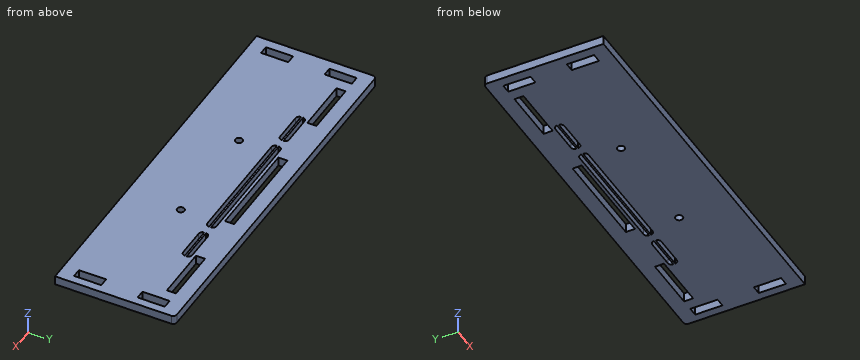
Autodesk Inventor part; units mm, degrees
ref_plane "YZ Plane" through (0, 0, 0) normal (1, 0, 0) x (0, 1, 0)
ref_plane "XZ Plane" through (0, 0, 0) normal (0, 1, 0) x (-1, 0, 0)
ref_plane "XY Plane" through (0, 0, 0) normal (0, 0, 1) x (1, 0, 0)
sketch "Sketch1" plane through (0, 0, 0) normal (0, 0, 1) x (1, 0, 0)
  line L0 (-104.38, -32.9991) -> (103.62, -32.9991)
  line L1 (-102.38, 33.0009) -> (101.62, 33.0009)
  line L2 (57.998, 18.2189) -> (41.998, 18.2189)
  line L3 (41.998, 13.2189) -> (57.998, 13.2189)
  line L4 (-58.002, 18.2189) -> (-42.002, 18.2189)
  line L5 (-42.002, 13.2189) -> (-58.002, 13.2189)
  line L6 (32.998, 18.2189) -> (-33.002, 18.2189)
  line L7 (-33.002, 13.2189) -> (32.998, 13.2189)
  arc A0 (34.998, 16.2189) -> (32.998, 18.2189) centre (32.998, 16.2189) ccw
  arc A1 (-35.002, 15.2189) -> (-33.002, 13.2189) centre (-33.002, 15.2189) ccw
  arc A2 (-33.002, 18.2189) -> (-35.002, 16.2189) centre (-33.002, 16.2189) ccw
  arc A3 (-40.002, 16.2189) -> (-42.002, 18.2189) centre (-42.002, 16.2189) ccw
  arc A4 (-42.002, 13.2189) -> (-40.002, 15.2189) centre (-42.002, 15.2189) ccw
  arc A5 (-60.002, 15.2189) -> (-58.002, 13.2189) centre (-58.002, 15.2189) ccw
  arc A6 (-58.002, 18.2189) -> (-60.002, 16.2189) centre (-58.002, 16.2189) ccw
  arc A7 (39.998, 15.2189) -> (41.998, 13.2189) centre (41.998, 15.2189) ccw
  arc A8 (41.998, 18.2189) -> (39.998, 16.2189) centre (41.998, 16.2189) ccw
  arc A9 (59.998, 16.2189) -> (57.998, 18.2189) centre (57.998, 16.2189) ccw
  arc A10 (57.998, 13.2189) -> (59.998, 15.2189) centre (57.998, 15.2189) ccw
  arc A11 (32.998, 13.2189) -> (34.998, 15.2189) centre (32.998, 15.2189) ccw
  line L8 (59.998, 16.2189) -> (39.998, 16.2189)
  line L9 (39.998, 15.2189) -> (59.998, 15.2189)
  line L10 (34.998, 16.2189) -> (-35.002, 16.2189)
  line L11 (-35.002, 15.2189) -> (34.998, 15.2189)
  line L12 (-40.002, 16.2189) -> (-60.002, 16.2189)
  line L13 (-60.002, 15.2189) -> (-40.002, 15.2189)
  circle A12 centre (-30.002, -2.9991) radius 2
  circle A13 centre (29.998, -2.9991) radius 2
  line L14 (-104.38, 31.0009) -> (-104.38, -32.9991)
  line L15 (103.62, 31.0009) -> (103.62, -32.9991)
  arc A14 (-102.38, 33.0009) -> (-104.38, 31.0009) centre (-102.38, 31.0009) ccw
  arc A15 (103.62, 31.0009) -> (101.62, 33.0009) centre (101.62, 31.0009) ccw
  line L16 (93.998, -24.9998) -> (93.998, -10.0006)
  line L17 (93.998, -10.0006) -> (98.998, -10.0006)
  line L18 (98.998, -24.9998) -> (98.998, -10.0006)
  line L19 (93.998, -24.9998) -> (98.998, -24.9998)
  line L20 (93.998, 9.9994) -> (93.998, 25.0009)
  line L21 (93.998, 25.0009) -> (98.998, 25.0009)
  line L22 (98.998, 9.9994) -> (98.998, 25.0009)
  line L23 (93.998, 9.9994) -> (98.998, 9.9994)
  line L24 (87.498, 20.0009) -> (57.498, 20.0009)
  line L25 (57.498, 20.0009) -> (57.498, 25.0009)
  line L26 (87.498, 25.0009) -> (57.498, 25.0009)
  line L27 (87.498, 20.0009) -> (87.498, 25.0009)
  line L28 (27.498, 20.0009) -> (-27.502, 20.0009)
  line L29 (-27.502, 20.0009) -> (-27.502, 25.0009)
  line L30 (27.498, 25.0009) -> (-27.502, 25.0009)
  line L31 (27.498, 20.0009) -> (27.498, 25.0009)
  line L32 (-57.502, 20.0009) -> (-87.502, 20.0009)
  line L33 (-87.502, 20.0009) -> (-87.502, 25.0009)
  line L34 (-57.502, 25.0009) -> (-87.502, 25.0009)
  line L35 (-57.502, 20.0009) -> (-57.502, 25.0009)
  line L36 (-99.002, 9.9994) -> (-99.002, 25.0009)
  line L37 (-99.002, 25.0009) -> (-94.002, 25.0009)
  line L38 (-94.002, 9.9994) -> (-94.002, 25.0009)
  line L39 (-99.002, 9.9994) -> (-94.002, 9.9994)
  line L40 (-99.002, -24.9998) -> (-99.002, -10.0006)
  line L41 (-99.002, -10.0006) -> (-94.002, -10.0006)
  line L42 (-94.002, -24.9998) -> (-94.002, -10.0006)
  line L43 (-99.002, -24.9998) -> (-94.002, -24.9998)
  point P0 (59.998, 18.2189)
  point P1 (59.998, 13.2189)
  point P2 (-40.002, 15.2189)
  point P3 (-60.002, 16.2189)
  point P4 (59.998, 15.2189)
  point P5 (34.998, 15.2189)
  point P6 (-35.002, 16.2189)
  point P7 (-0.002, -3)
extrude "Extrusion1" add sketch "Sketch1" along normal blind 5
properties part number "case bottom front" material "Nylon, molybdenum disulphide"
The model under review builds one solid part; all positions refer to its coordinate system, in mm. Round coordinates to 2 decimals unless told otherwise and drop trailing zeros. Order: outer loops, then holes, each group sorted by start corner. A loop starts at its lowest first (then second) coordinate and runs counter-clockwise, first axis right, second up. Notation, with made-up numbers: (23.5, -19.5) -> (32.5, -19.5) arc R20 cw to (32.5, -3.5) -> close; hole circle Ø9 at (56.25, 59.25). An arc over 180 degrees is marked (long way). Use a Markdown table: item, result.
Q1. We need section D-D on x = -74. Write out the cut boundary in (y, z), then the cut area to 3 significant figures.
Values:
| item | result |
|---|---|
| outline | (-33, 0) -> (20, 0) -> (20, 5) -> (-33, 5) -> close; (25, 0) -> (33, 0) -> (33, 5) -> (25, 5) -> close |
| area | 305 mm^2 |
Q2. We need section B-B on y = 23. Write out the cut boundary in (x, z), then the cut area to 3 significant figures.
Values:
| item | result |
|---|---|
| outline | (-104.38, 0) -> (-99, 0) -> (-99, 5) -> (-104.38, 5) -> close; (-94, 0) -> (-87.5, 0) -> (-87.5, 5) -> (-94, 5) -> close; (-57.5, 0) -> (-27.5, 0) -> (-27.5, 5) -> (-57.5, 5) -> close; (27.5, 0) -> (57.5, 0) -> (57.5, 5) -> (27.5, 5) -> close; (87.5, 0) -> (94, 0) -> (94, 5) -> (87.5, 5) -> close; (99, 0) -> (103.62, 0) -> (103.62, 5) -> (99, 5) -> close |
| area | 415 mm^2 |
Q3. We need section A-A on x = 48.5. Write out the cut boundary in (y, z), then the cut area to 3 significant figures.
Values:
| item | result |
|---|---|
| outline | (-33, 0) -> (13.22, 0) -> (13.22, 5) -> (-33, 5) -> close; (15.22, 0) -> (16.22, 0) -> (16.22, 5) -> (15.22, 5) -> close; (18.22, 0) -> (33, 0) -> (33, 5) -> (18.22, 5) -> close |
| area | 310 mm^2 |
Q4. We need section C-C on y = -22. Write out the cut boundary in (x, z), then the cut area to 3 significant figures.
Values:
| item | result |
|---|---|
| outline | (-104.38, 0) -> (-99, 0) -> (-99, 5) -> (-104.38, 5) -> close; (-94, 0) -> (94, 0) -> (94, 5) -> (-94, 5) -> close; (99, 0) -> (103.62, 0) -> (103.62, 5) -> (99, 5) -> close |
| area | 990 mm^2 |
Q5. For line 1 (X direction, y = -20.5, z = 0.65); line 2 (X direction, y = 15, z = 0.4); line 3 (X direction, y = -3, z = 2.05), list the stretches that pass through material, from the lowest coordinate up.
Values:
| item | result |
|---|---|
| line 1 | x = -104.38 to -99, -94 to 94, 99 to 103.62 |
| line 2 | x = -104.38 to -99, -94 to -59.99, -40.01 to -34.99, 34.99 to 40.01, 59.99 to 94, 99 to 103.62 |
| line 3 | x = -104.38 to -32, -28 to 28, 32 to 103.62 |
